Check sheet for the modelled part. Datum: model origin and axes. Units: mm. Face numbers are marked on the shaded views. Round coordinates to 2 decimals unless told otherwise and drop trailing zeros. Order: outer loops, then holes, each group sorted by start corner. A loop starts at its lowest first (then second) coordinate and runs counter-clockwise, first axis right, second up.
(1) Sectioned sample at A-A, the plane z = -12. Enter the section's corners in (x, y), and give its area (3 significant figures).
(2) Depth check by flat-ended pin: pin 1 (6 mm diameter, centred on x = -38, y = -38.5, fed in from -Z). Enter the tip coordinate at first touch or a pass-through.
(3) Mould release check, pull along Y, two halves, no side actions. Record for the marked faces 1, 2, 3 and 4: released by +Y, released by -Y, zero draft, split by the parting line, or undercut.
(4) Sectioned sample at C-C, the plane y = -18. Enter the section's corners in (x, z), and give its area (3 significant figures).
(5) Sectioned sample at B-B, the plane x = 33. Enter the section's corners in (y, z), and give its area (3 significant figures).
(6) Thickness scan on probe 1 along Y at (x, z) = (8.5, 23.5); probe 2 along X at (y, z) = (-28.5, -12); probe 3 along Z at (x, y) = (20, -18.5). Record the ranges inside material, lowest first.
```python
from build123d import *

# Parameters (mm, degrees)
F0_W         = 126.0307952762
F0_H         = 54.4428955764
F1_DEPTH     = 50.8
F2_R         = 5.08
F3_T1_DEPTH  = 62.0628955764
F3_S5_W      = 5.08
F3_S5_H      = 5.08
F3_T6_DEPTH  = 5.08
F3_S11_W     = 5.08
F3_S11_H     = 5.08
F3_T12_DEPTH = 5.08
F4_DEPTH     = 47.752


# Not quite as in the source:
# - a fillet or chamfer that OpenCascade refuses, or shapes differently, is made with other operations: its cross-section is extruded or revolved along the edge and cut away or added


with BuildPart() as f1:
    # F0 (on Front) → F1 (new body)
    with BuildSketch(Plane.XZ):
        with Locations((3.3086873591, 6.0157896951)):
            Rectangle(F0_W, F0_H)
    extrude(amount=F1_DEPTH)

    # F2
    f2_edges = [f1.edges().sort_by_distance(p)[0] for p in [
        (66.324085, -50.8, 6.01579),
        (-59.70671, -50.8, 6.01579),
        (3.308687, -50.8, -21.205658),
        (-59.70671, -25.4, -21.205658),
        (66.324085, -25.4, -21.205658),
        (3.308687, 0, -21.205658),
    ]]
    fillet(f2_edges, radius=F2_R)

    # F3: fillet of radius 5.08 on 2 edges, made by hand

    # F3_s2 → F3_t1 (cut)
    with BuildSketch(Plane.XY.offset(-16.1256580931)):
        with BuildLine():
            ThreePointArc((66.3240849972, -5.08), (64.8361874456, -1.4878975516), (61.2440849972, 0))
            Line((61.2440849972, 0), (66.3240849972, 0))
            Line((66.3240849972, 0), (66.3240849972, -5.08))
        make_face()
        with BuildLine():
            ThreePointArc((-54.626710279, 0), (-58.2188127274, -1.4878975516), (-59.706710279, -5.08))
            Line((-59.706710279, -5.08), (-59.706710279, 0))
            Line((-59.706710279, 0), (-54.626710279, 0))
        make_face()
    extrude(amount=F3_T1_DEPTH, mode=Mode.SUBTRACT)


with BuildPart() as f3_tool4:
    # F3_s5 → F3_t6 (new body)
    with BuildSketch(Plane.XZ.offset(5.08)):
        with Locations((-57.166710279, -18.6656580931)):
            Rectangle(F3_S5_W, F3_S5_H)
    extrude(amount=-F3_T6_DEPTH)

    # F3_s7 → F3_t8 (revolve, cut)
    with BuildSketch(Plane(origin=(-54.626710279, -5.08, -16.1256580931), x_dir=(0.7071067812, 0, 0.7071067812), z_dir=(-0.7071067812, 0, 0.7071067812))):
        with BuildLine():
            ThreePointArc((0, -5.08), (5.08, 0), (0, 5.08))
            Line((0, 5.08), (0, -5.08))
        make_face()
    revolve(axis=Axis((-54.626710279, -5.08, -16.1256580931), (0, 1, 0)), mode=Mode.SUBTRACT)


with BuildPart() as f1_1:
    add(f1.part)

    # F3_t3: cut F3_tool4
    add(f3_tool4.part, mode=Mode.SUBTRACT)


with BuildPart() as f3_tool10:
    # F3_s11 → F3_t12 (new body)
    with BuildSketch(Plane.YZ.offset(61.2440849972)):
        with Locations((-2.54, -18.6656580931)):
            Rectangle(F3_S11_W, F3_S11_H)
    extrude(amount=F3_T12_DEPTH)

    # F3_s13 → F3_t14 (revolve, cut)
    with BuildSketch(Plane(origin=(61.2440849972, -5.08, -16.1256580931), x_dir=(0, -0.7071067812, 0.7071067812), z_dir=(0, 0.7071067812, 0.7071067812))):
        with BuildLine():
            ThreePointArc((0, -5.08), (5.08, 0), (0, 5.08))
            Line((0, 5.08), (0, -5.08))
        make_face()
    revolve(axis=Axis((61.2440849972, -5.08, -16.1256580931), (1, 0, 0)), mode=Mode.SUBTRACT)


with BuildPart() as f1_2:
    add(f1_1.part)

    # F3_t9: cut F3_tool10
    add(f3_tool10.part, mode=Mode.SUBTRACT)

    # F4 (cut): a face of the model
    f4_faces = [f1_2.faces().sort_by_distance(p)[0] for p in [
        (3.3086873591, -25.4, -21.2056580931),
    ]]
    extrude(f4_faces, amount=-F4_DEPTH, mode=Mode.SUBTRACT)


solid = f1_2.part
```
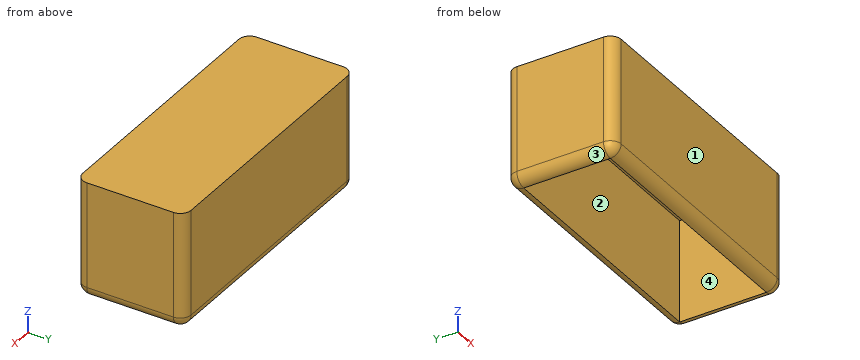
Derived:
1. outline: (-59.71, -45.72) arc R5.08 ccw to (-54.63, -50.8) - (61.24, -50.8) arc R5.08 ccw to (66.32, -45.72) - (66.32, -5.08) arc R5.08 ccw to (61.24, 0) - (-54.63, 0) arc R5.08 ccw to (-59.71, -5.08) - close; hole (-54.63, -45.72) - (61.24, -45.72) - (61.24, -5.08) - (-54.63, -5.08) - close
1. area: 1,670 mm2
2. pin 1: stops at z = 26.55
3. face 1: released by -Y
3. face 2: undercut
3. face 3: zero draft
3. face 4: undercut
4. outline: (-59.71, -16.13) arc R5.08 ccw to (-54.63, -21.21) - (-54.63, 26.55) - (61.24, 26.55) - (61.24, -21.21) arc R5.08 ccw to (66.32, -16.13) - (66.32, 33.24) - (-59.71, 33.24) - close
4. area: 1,320 mm2
5. outline: (-50.8, -16.13) arc R5.08 ccw to (-45.72, -21.21) - (-45.72, 26.55) - (-5.08, 26.55) - (-5.08, -21.21) arc R5.08 ccw to (0, -16.13) - (0, 33.24) - (-50.8, 33.24) - close
5. area: 814 mm2
6. probe 1: y = -50.8 to -45.72, -5.08 to 0
6. probe 2: x = -59.71 to -54.63, 61.24 to 66.32
6. probe 3: z = 26.55 to 33.24
